from build123d import *

# Parameters (mm, degrees)
F0_W     = 21.2045684457
F0_H     = 21.2045684457
F0_H_2   = 23.2402067631
F1_DEPTH = 25.4
F2_W     = 12.7
F2_H     = 27.5493436545
F3_DEPTH = 101.6
F4_W     = 14.3764
F4_H     = 41.4685436545
F5_DEPTH = 254
F7_DEPTH = 14.3764
F8_R     = 5.08


with BuildPart() as f1:
    # F0 (on Front) → F1 (new body)
    with BuildSketch(Plane.XZ):
        with Locations((10.6022842228, 33.842490986)):
            Rectangle(F0_W, F0_H)
        with Locations((10.6022842228, -10.6022842228)):
            Rectangle(F0_W, F0_H)
        with Locations((10.6022842228, 11.6201033816)):
            Rectangle(F0_W, F0_H_2)
    extrude(amount=F1_DEPTH)

    # F2 (on face) → F3 (join)
    with BuildSketch(Plane.YZ.offset(21.2045684457)):
        with Locations((-12.7, 11.6201033816)):
            Rectangle(F2_W, F2_H)
    extrude(amount=F3_DEPTH)

    # F4 (on face) → F5 (join)
    with BuildSketch(Plane(origin=(0, 0, 0), x_dir=(0, -1, 0), z_dir=(-1, 0, 0))):
        with Locations((12.7, 11.6201033816)):
            Rectangle(F4_W, F4_H)
    extrude(amount=F5_DEPTH)

    # F6 (on face) → F7 (join)
    with BuildSketch(Plane.XZ.offset(19.8882)):
        Polygon((-254, -9.1141684457), (-254, 32.3543752088), (-325.8476853371, 11.6201033816), align=None)
    extrude(amount=-F7_DEPTH)

    # F8
    f8_edges = [f1.edges().sort_by_distance(p)[0] for p in [
        (21.204568, -25.4, 11.620103),
        (0, -25.4, 11.620103),
        (0, 0, 11.620103),
        (21.204568, 0, 11.620103),
        (10.602284, -25.4, 44.444775),
        (21.204568, -12.7, 44.444775),
        (10.602284, 0, 44.444775),
        (0, -12.7, 44.444775),
        (10.602284, -25.4, -21.204568),
        (21.204568, -12.7, -21.204568),
        (0, -12.7, -21.204568),
        (10.602284, 0, -21.204568),
        (122.804568, -19.05, 11.620103),
        (122.804568, -6.35, 11.620103),
        (122.804568, -12.7, -2.154568),
        (122.804568, -12.7, 25.394775),
        (72.004568, -19.05, 25.394775),
        (72.004568, -6.35, 25.394775),
        (72.004568, -19.05, -2.154568),
        (72.004568, -6.35, -2.154568),
    ]]
    fillet(f8_edges, radius=F8_R)


solid = f1.part
Verification items for the finished model (mm, model axes). A direction names the side the tool comes from. Round coordinates to 2 decimals unless told otherwise and drop trailing zeros. Order: outer loops, then holes, each group sorted by start corner. A loop starts at its lowest first (then second) coordinate and runs counter-clockwise, first axis right, second up.
1. Section check A-A on x = 74.5. Record the cut outline in (y, z), then the cut area to 3 significant figures.
Final values:
outline: (-19.05, 2.93) arc R5.08 ccw to (-13.97, -2.15) - (-11.43, -2.15) arc R5.08 ccw to (-6.35, 2.93) - (-6.35, 20.31) arc R5.08 ccw to (-11.43, 25.39) - (-13.97, 25.39) arc R5.08 ccw to (-19.05, 20.31) - close
area: 328 mm2
2. Access from +Z, -Z, +X, -X, +Y, -Y to the whole of each face (thin tool, end or side, straight path). Record for faces 1 (the flat face through (21.205, -6, 11)), 2 (the flat face through (69, -6.35, 11)), 3 (the flat face through (-125, -13, -9.114)).
Final values:
face 1: +X
face 2: +Z, -Z, +X, +Y
face 3: -Z, -X, +Y, -Y
3. Thickness scan on L1, parallel to Z at x = -146.5, y = -7; L2, parallel to Z at x = 75.5, y = -12.25; L3, parallel to Y at x = -135, z = 8. Record the ranges inside material, lowest first.
Final values:
L1: z = -9.11 to 32.35
L2: z = -2.15 to 25.39
L3: y = -19.89 to -5.51
4. Section check C-C on x = -293.5. Record the cut outline in (y, z) (3 decimals), then the cut area to 3 significant figures.
Final values:
outline: (-19.888, 2.285) - (-5.512, 2.285) - (-5.512, 20.955) - (-19.888, 20.955) - close
area: 268 mm2
5. Section check B-B on x = -139.5. Record the cut outline in (y, z).
Final values:
outline: (-19.89, -9.11) - (-5.51, -9.11) - (-5.51, 32.35) - (-19.89, 32.35) - close
6. Go/stop test with flat-tipped pins: P1, Ø4, axis at x = 3, z = 5, coming from the +Y side; P2, Ø4.5, axis at x = -108.5, y = -11, coming from the +Z side; P3, Ø14, axis at x = 92, z = 12.5, coming from the +Y side; P4, Ø2, axis at x = -136, z = -7.5, coming from the -Y side. Record where each tip stops, or that it passes through.
Final values:
P1: stops at y = 0
P2: stops at z = 32.35
P3: stops at y = -6.35
P4: stops at y = -19.89
